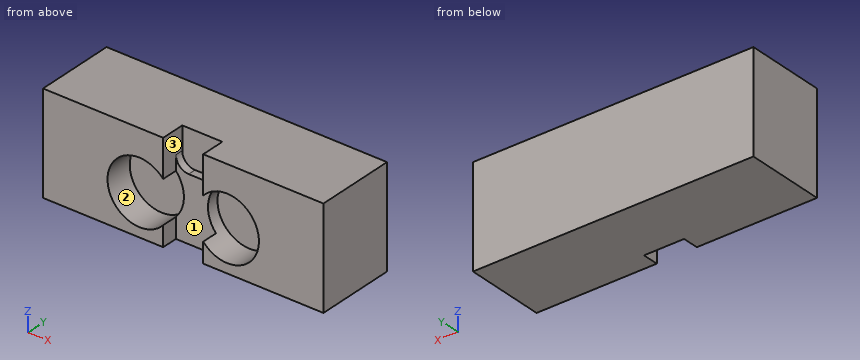
from build123d import *

# Parameters (mm, degrees)
SKETCH1_W           = 70
SKETCH1_H           = 25
BOSS_EXTRUDE1_DEPTH = 20
SKETCH2_R           = 7.95
CUT_EXTRUDE1_DEPTH  = 7
SKETCH3_W           = 10
SKETCH3_H           = 25
CUT_EXTRUDE2_DEPTH  = 4
SKETCH7_W           = 10
SKETCH7_H           = 9
CUT_EXTRUDE3_DEPTH  = 6
FILLET1_R           = 3.2


with BuildPart() as part:
    # Sketch1 → Boss-Extrude1 (new body)
    with BuildSketch(Plane(origin=(0, 0, 0), x_dir=(1, 0, 0), z_dir=(0, 1, 0))):
        Rectangle(SKETCH1_W, SKETCH1_H)
    extrude(amount=-BOSS_EXTRUDE1_DEPTH)

    # Sketch2 → Cut-Extrude1 (cut)
    with BuildSketch(Plane.XZ.offset(20)):
        with Locations(Location((-10.95, -2.198838129, 0), (0, 0, 270))):
            Circle(SKETCH2_R)
        with Locations(Location((10.95, -2.198838129, 0), (0, 0, 270))):
            Circle(SKETCH2_R)
    extrude(amount=-CUT_EXTRUDE1_DEPTH, mode=Mode.SUBTRACT)

    # Sketch3 → Cut-Extrude2 (cut)
    with BuildSketch(Plane.XZ.offset(20)):
        Rectangle(SKETCH3_W, SKETCH3_H)
    extrude(amount=-CUT_EXTRUDE2_DEPTH, mode=Mode.SUBTRACT)

    # Sketch7 → Cut-Extrude3 (cut)
    with BuildSketch(Plane.XZ.offset(20)):
        with Locations((0, 8)):
            Rectangle(SKETCH7_W, SKETCH7_H)
    extrude(amount=-CUT_EXTRUDE3_DEPTH, mode=Mode.SUBTRACT)

    # Fillet1
    fillet1_edges = [part.edges().sort_by_distance(p)[0] for p in [
        (5, -15, 3.5),
        (-5, -15, 3.5),
    ]]
    fillet(fillet1_edges, radius=FILLET1_R)


solid = part.part
Model file for the job. Use its own axes, mm. Face numbers are marked on the shaded views. A direction names the side the tool comes from. Give positions to 0.01 mm unless a question says otherwise; leave off trailing zeros. Loops run counter-clockwise (first coordinate to the right, second up) from the corner with the lowest first, then second, coordinate; pieces in that order, holes last.
Item 1: Slice it at C-C (z = -6). Write the cut outline in (x, y), plus the area to 3 significant figures.
Check values:
outline: (-35, -20) - (-17.93, -20) - (-17.93, -13) - (-3.97, -13) - (-3.97, -16) - (3.97, -16) - (3.97, -13) - (17.93, -13) - (17.93, -20) - (35, -20) - (35, 0) - (-35, 0) - close
area: 1,170 mm2
Item 2: Drop flat-ended pins along their axis: P1, Ø9.5, axis at x = 10.95, z = -2.2, coming from the -Y side; P2, Ø5, axis at x = 2, z = -1, coming from the -Y side; P3, Ø0.6, axis at x = 0.5, y = -15, coming from the +Z side; P4, Ø12.5, axis at x = -7.5, z = -0.5, coming from the -Y side. Give the stop position or say it passes through.
Check values:
P1: stops at y = -13
P2: stops at y = -16
P3: stops at z = 3.5
P4: stops at y = -20
Item 3: Slice it at A-A (z = 7.5). Write the cut outline in (x, y), plus the area to 3 significant figures.
Check values:
outline: (-35, -20) - (-5, -20) - (-5, -14) - (5, -14) - (5, -20) - (35, -20) - (35, 0) - (-35, 0) - close
area: 1,340 mm2
Item 4: Which spindle directions (+Z, -Z, +X, -X, +Y, -Y) get a long thin tool onto all of the face, cutting with end or side? Do the marked faces 1, 2 and 3. Say none if no direction does.
Check values:
face 1: +Z, -Z, -Y
face 2: -Y
face 3: +Z, -Y
Item 5: Drill centre lines: line 1 along Z through (x, y) = (10.95, -18); line 2 along Y through (x, z) = (3, -6); line 3 along Y through (x, z) = (-4, 7.5). Where is each one in solid material? Low to high.
Check values:
line 1: z = -12.5 to -10.15, 5.75 to 12.5
line 2: y = -16 to 0
line 3: y = -14 to 0
Item 6: Slice it at D-D (z = -0.5). Write the cut outline in (x, y), plus the area to 3 significant figures.
Check values:
outline: (-35, -20) - (-18.72, -20) - (-18.72, -13) - (-3.18, -13) - (-3.18, -16) - (3.18, -16) - (3.18, -13) - (18.72, -13) - (18.72, -20) - (35, -20) - (35, 0) - (-35, 0) - close
area: 1,160 mm2
Item 7: Slice it at B-B (x = -10.95). Write the cut outline in (y, z).
Check values:
outline: (-20, -12.5) - (0, -12.5) - (0, 12.5) - (-20, 12.5) - (-20, 5.75) - (-13, 5.75) - (-13, -10.15) - (-20, -10.15) - close
